```python
from build123d import *

# Parameters (mm, degrees)
F0_R     = 1.1684
F0_R_2   = 2.413
F0_R_3   = 1.143
F0_R_4   = 0.79375
F1_DEPTH = 2.38125
F2_R     = 0.8128


with BuildPart() as f1:
    # F0 (on Top) → F1 (new body)
    with BuildSketch(Plane.XY):
        with BuildLine():
            Line((31.5976, 7.6708), (0, 7.6708))
            Line((0, 7.6708), (-31.5976, 7.6708))
            ThreePointArc((-31.5976, 7.6708), (-39.240111, 0.658177), (-32.909099, -7.557853))
            Line((-32.909099, -7.557853), (-6.35, -12.1666))
            Line((-6.35, -12.1666), (6.35, -12.1666))
            Line((6.35, -12.1666), (32.909099, -7.557853))
            ThreePointArc((32.909099, -7.557853), (39.240111, 0.658177), (31.5976, 7.6708))
        make_face()
        with Locations((-3.673187, -9.745723)):
            Circle(F0_R, mode=Mode.SUBTRACT)
        with Locations((3.673187, -9.745723)):
            Circle(F0_R, mode=Mode.SUBTRACT)
        with Locations((0, -8.259213)):
            Circle(F0_R, mode=Mode.SUBTRACT)
        with Locations((-25.019, 0)):
            Circle(F0_R_2, mode=Mode.SUBTRACT)
        with Locations((-20.0152, 0)):
            Circle(F0_R_3, mode=Mode.SUBTRACT)
        with Locations((-36.0934, 0.5334)):
            Circle(F0_R_4, mode=Mode.SUBTRACT)
        with Locations((-15.0114, 0)):
            Circle(F0_R_2, mode=Mode.SUBTRACT)
        with Locations((-5.0038, 0)):
            Circle(F0_R_2, mode=Mode.SUBTRACT)
        with Locations((5.0038, 0)):
            Circle(F0_R_2, mode=Mode.SUBTRACT)
        with Locations((15.0114, 0)):
            Circle(F0_R_2, mode=Mode.SUBTRACT)
        with Locations((20.0152, 0)):
            Circle(F0_R_3, mode=Mode.SUBTRACT)
        with Locations((25.019, 0)):
            Circle(F0_R_2, mode=Mode.SUBTRACT)
        with Locations((36.0934, 0.5334)):
            Circle(F0_R_4, mode=Mode.SUBTRACT)
    extrude(amount=F1_DEPTH)

    # F2
    f2_edges = [f1.edges().sort_by_distance(p)[0] for p in [
        (-39.240111, 0.658177, 2.38125),
        (-19.629549, -9.862227, 2.38125),
        (0, -12.1666, 2.38125),
    ]]
    fillet(f2_edges, radius=F2_R)


solid = f1.part
```
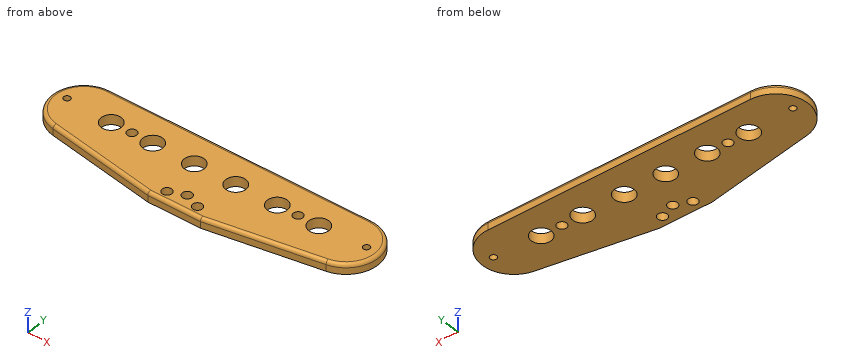
For this review, take the finished solid that the model builds, in its own axes (mm). Round coordinates to 2 decimals unless told otherwise and drop trailing zeros. Write each loop counter-clockwise with the first axis right and the second up, starting at its lowest first coordinate (ties: lowest second). Pieces come first, ordered by that corner, then holes. Notation, with made-up numbers: (-5, -9.5) - (9, -9.5) arc R19 ccw to (9, 16.5) - close; hole circle Ø1 at (75, 87.25). An arc over 180 degrees is marked (long way). Answer as a JSON object with one key per item and string values.
1. For pin 1 Ø5 at (x, y) = (4, -5) entering from -Z; pin 2 Ø4.5 at (x, y) = (-5, 0) entering from -Z, all flat-tipped, find the tip position at first contact; note any pin that passes through.
Response values:
{"pin 1": "stops at z = 0", "pin 2": "passes through"}
2. To check wall thickness, follow line 1 along Y through (x, z) = (13, 2.1); line 2 along Y through (x, z) = (36, 1.5); line 3 along Y through (x, z) = (11, 0.85). State the ranges of each line that lie inside material, in increasing order.
Response values:
{"line 1": "y = -10.81 to -1.33, 1.33 to 7.47", "line 2": "y = -6.28 to -0.25, 1.32 to 6.28", "line 3": "y = -11.36 to 7.67"}
3. We need section A-A on x = 0. Give the boundary of the cut face in (y, z), then the cut area to 3 significant figures.
Response values:
{"outline": "(-12.17, 0) - (-9.43, 0) - (-9.43, 2.38) - (-11.35, 2.38) arc R0.81 ccw to (-12.17, 1.57) - close; (-7.09, 0) - (7.67, 0) - (7.67, 1.57) arc R0.81 ccw to (6.86, 2.38) - (-7.09, 2.38) - close", "area": "41.4 mm2"}
4. We need section B-B on z = 0.55. Count the separate pieces of the cut face and the enclosed holes in it, then the cut area to 3 significant figures.
Response values:
{"separate pieces": "1", "enclosed holes": "13", "area": "1,190 mm2"}
